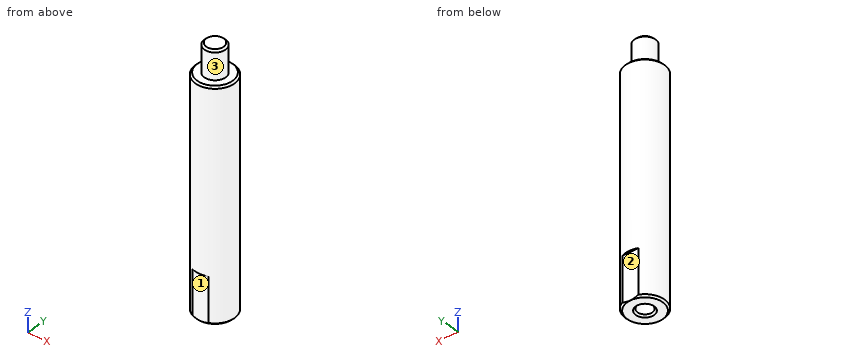
from build123d import *

# Parameters (mm, degrees)
SKETCH_1_R             = 5.5
EXTRUDE_1_DEPTH        = 64
CHAMFER_1_SIZE         = 0.5
SKETCH_2_R             = 3.3
EXTRUDE_2_DEPTH        = 8
HOLE_WIZARD_M5_1_D     = 4.2
HOLE_WIZARD_M5_1_DEPTH = 12.4
HOLE_WIZARD_M5_1_TIP   = 1.2618073
CHAMFER_3_SIZE         = 0.5
SKETCH_6_W             = 10
SKETCH_6_H             = 3
CUT_EXTRUDE_1_DEPTH    = 13


# Read off the part's stored shape, not the designer's step: M6 机械螺纹 螺柱1
with BuildPart() as part:
    # 草图1 → 拉伸1 (new body)
    with BuildSketch(Plane.XY):
        Circle(SKETCH_1_R)
    extrude(amount=EXTRUDE_1_DEPTH)

    # 倒角1
    chamfer_1_edges = [part.edges().sort_by_distance(p)[0] for p in [
        (-5.5, 0, 0),
        (-5.5, 0, 64),
    ]]
    chamfer(chamfer_1_edges, length=CHAMFER_1_SIZE)

    # 草图2 → 拉伸2 (add)
    with BuildSketch(Plane.XY.offset(64)):
        Circle(SKETCH_2_R)
    extrude(amount=EXTRUDE_2_DEPTH)

    # M5 螺纹孔1
    with Locations(Plane(origin=(0, 0, 0), x_dir=(-1, 0, 0), z_dir=(0, 0, -1))):
        with Locations((0, 0)):
            Hole(HOLE_WIZARD_M5_1_D / 2, depth=HOLE_WIZARD_M5_1_DEPTH)
            with Locations((0, 0, -(HOLE_WIZARD_M5_1_DEPTH + HOLE_WIZARD_M5_1_TIP / 2))):  # 118° drill point
                Cone(0, HOLE_WIZARD_M5_1_D / 2, HOLE_WIZARD_M5_1_TIP, mode=Mode.SUBTRACT)

    # 倒角3
    chamfer_3_edges = [part.edges().sort_by_distance(p)[0] for p in [
        (-2.1, 0, 0),
    ]]
    chamfer(chamfer_3_edges, length=CHAMFER_3_SIZE)

    # 草图6 → 切除-拉伸1 (cut)
    with BuildSketch(Plane(origin=(0, 0, 0), x_dir=(-1, 0, 0), z_dir=(0, 0, -1))):
        with Locations((0, 6.5)):
            Rectangle(SKETCH_6_W, SKETCH_6_H)
        with Locations((0, -6.5)):
            Rectangle(SKETCH_6_W, SKETCH_6_H)
    extrude(amount=-CUT_EXTRUDE_1_DEPTH, mode=Mode.SUBTRACT)

    # M6 机械螺纹 螺柱1 outline → M6 机械螺纹 螺柱1 (revolve, cut)
    with BuildSketch(Plane.XZ):
        Polygon((3.3, 72), (2.4585, 72), (3, 71.4585), (3, 64), (3.3, 64), align=None)
    revolve(axis=Axis((0, 0, 0), (0, 0, 1)), mode=Mode.SUBTRACT)


solid = part.part
Here's how the part is built. I have some questions about the finished solid (model axes, mm). Face numbers are marked on the shaded views. A direction names the side the tool comes from. Coordinates: 2 decimals unless noted, no trailing zeros. Order: outer loops, then holes, each group sorted by start corner. A loop starts at its lowest first (then second) coordinate and runs counter-clockwise, first axis right, second up. Notation, with made-up numbers: (19.25, -6.75) -> (69.25, -6.75) arc R22 ccw to (69.25, 11.25) -> close; hole circle Ø7 at (72.5, 60). An arc over 180 degrees is marked (long way). Answer in a Markdown table with one row per item.
(1) Will these pins go through, and if not, where does the flat tip stop? pin 1 Ø0.6 at (x, y) = (0.5, -5.5) entering from -Z; pin 2 Ø3 at (y, z) = (4, 21) entering from +X; pin 3 Ø1.5 at (x, z) = (-2.5, 60.5) entering from +Y; pin 4 Ø6.5 at (x, y) = (0, 0) entering from -Z.
Answer key:
| item | result |
|---|---|
| pin 1 | z = 13 |
| pin 2 | x = 4.9 |
| pin 3 | y = 5.21 |
| pin 4 | z = 0 |
(2) I want a section at B-B on z = 66. List the corners of the cut face in (x, y) for me.
Answer key:
| item | result |
|---|---|
| outline | circle Ø6 at (0, 0) |
(3) I want a section at C-C on z = 52. List the corners of the cut face in (x, y) for me.
Answer key:
| item | result |
|---|---|
| outline | circle Ø11 at (0, 0) |
(4) On a 3-axis mill with a long thin cutter (end or side, diameter ignored), from which of +Z, -Z, +X, -X, +Y, -Y can I reach the whole of each face in a straight line? I mean the marked faces 1, 2 and 3. Say none if no direction works.
Answer key:
| item | result |
|---|---|
| face 1 | -Z, +X, -X, -Y |
| face 2 | -Z, +X, -X, +Y |
| face 3 | +Z |
(5) I want a section at A-A on z = 10. List the corners of the cut face in (x, y) for me, then the cut area to 3 significant figures.
Answer key:
| item | result |
|---|---|
| outline | (-2.29, -5) -> (2.29, -5) arc R5.5 ccw to (2.29, 5) -> (-2.29, 5) arc R5.5 ccw to start; hole circle Ø4.2 at (0, 0) |
| area | 78.1 mm^2 |
(6) Please list where these lines run through material, in increasing order: probe 1 along Y at (x, z) = (0, 4.5); probe 2 along X at (y, z) = (0, 10.25); probe 3 along Z at (x, y) = (4, -2.25).
Answer key:
| item | result |
|---|---|
| probe 1 | -5 to -2.1, 2.1 to 5 |
| probe 2 | -5.5 to -2.1, 2.1 to 5.5 |
| probe 3 | 0 to 64 |
